For this review, take the finished solid that the model builds, in its own axes (mm). Coordinates: 2 decimals unless noted, no trailing zeros. Order: outer loops, then holes, each group sorted by start corner. A loop starts at its lowest first (then second) coordinate and runs counter-clockwise, first axis right, second up. Notation, with made-up numbers: (13, -36) -> (60, -36) arc R8 cw to (60, -28) -> close; hole circle Ø5 at (73, -24). An arc over 180 degrees is marked (long way). Answer as a JSON object with one key per item and string values. Group by question number.
1) Wall thickness on L1, parallel to Z at x = 10.05, y = 16; L2, parallel to Y at x = 6.85, z = 109.5; L3, parallel to Y at x = 9.05, z = 112: over which ranges is each line inside the solid? List them lowest first.
2) Add section A-A, the plane y = 57.15. Write out the cut boundary in (x, z).
3) Add section B-B, the plane z = 0. Write out the cut boundary in (x, y).
4) Add section C-C, the plane x = 11.3. Count the separate pieces of the cut face and the enclosed holes in it, then the cut area to 3 significant figures.
5) Add section D-D, the plane y = 160. Write out the cut boundary in (x, z).
6) For pin 1 (2 mm diameter, centred on x = 10, y = 144, fed in from -Z); pin 2 (3 mm diameter, centred on x = 10.5, z = 36.5, fed in from -Y); pin 3 (3 mm diameter, centred on x = 9.5, y = 136.5, fed in from -Z), all flat-tipped, find the tip position at first contact; note any pin that passes through.
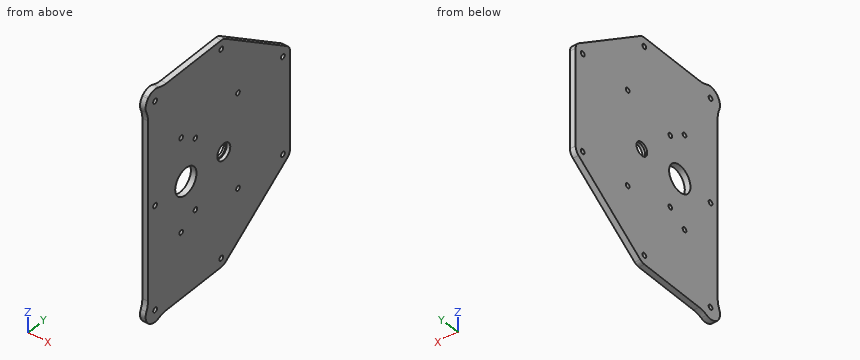
from build123d import *
from build123d.topology import SkipClean

# Parameters (mm, degrees)
ANGLEDBALLAST_DECKFRONT_OUTLINE_R = 2.5527
ANGLEDBALLAST_DECKFRONT_DEPTH     = 6.35
SKETCH1_R                         = 2.5527
BOSS_EXTRUDE1_DEPTH               = 5.9944
SKETCH2_R                         = 7.14375
SKETCH2_R_2                       = 14.2875
CUT_EXTRUDE1_DEPTH                = 344.885135927
F_10_CLEARANCE_HOLE1_AT_2_COUNT   = 2
F_10_CLEARANCE_HOLE1_AT_2_PITCH   = 58.544107304
F_10_CLEARANCE_HOLE1_AT_3_COUNT   = 2
F_10_CLEARANCE_HOLE1_AT_3_PITCH   = 105.685062805
F_10_CLEARANCE_HOLE1_AT_4_COUNT   = 2
F_10_CLEARANCE_HOLE1_AT_4_PITCH   = 76.2
F_10_CLEARANCE_HOLE1_AT_5_COUNT   = 2
F_10_CLEARANCE_HOLE1_AT_5_PITCH   = 90.539312574
F_10_CLEARANCE_HOLE1_AT_6_COUNT   = 2
F_10_CLEARANCE_HOLE1_AT_6_PITCH   = 22.719352983
SKETCH6_R                         = 12.7
SKETCH6_R_2                       = 2.5527
BOSS_EXTRUDE2_DEPTH               = 5.9944
FILLET1_R                         = 25.4
CUT_EXTRUDE2_DEPTH                = 233.633802265
FILLET2_R                         = 9.525
SKETCH8_R                         = 8.73125
CUT_EXTRUDE3_DEPTH                = 3.7846


# Read off the part's stored shape, not the designer's step: Surface Bodies1
with BuildPart() as part:
    # AngledBallast_DeckFront outline → AngledBallast_DeckFront (new body)
    with BuildSketch(Plane.YZ):
        Polygon((227.241295543, 95.25), (0, 257.81), (0, -257.81), (227.241295543, -95.25), align=None)
        with Locations((15.875, -111.125)):
            Circle(ANGLEDBALLAST_DECKFRONT_OUTLINE_R, mode=Mode.SUBTRACT)
        with Locations((104.656174089, -111.125)):
            Circle(ANGLEDBALLAST_DECKFRONT_OUTLINE_R, mode=Mode.SUBTRACT)
        with Locations((187.325, -51.986786112)):
            Circle(ANGLEDBALLAST_DECKFRONT_OUTLINE_R, mode=Mode.SUBTRACT)
        with Locations((15.875, 0)):
            Circle(ANGLEDBALLAST_DECKFRONT_OUTLINE_R, mode=Mode.SUBTRACT)
        with Locations((15.875, 111.125)):
            Circle(ANGLEDBALLAST_DECKFRONT_OUTLINE_R, mode=Mode.SUBTRACT)
        Polygon((101.6, -101.6), (25.4, -101.6), (25.4, 101.6), (101.6, 101.6), (177.8, 47.089344398), (177.8, -47.089344398), align=None, mode=Mode.SUBTRACT)
        with Locations((104.656174089, 111.125)):
            Circle(ANGLEDBALLAST_DECKFRONT_OUTLINE_R, mode=Mode.SUBTRACT)
        with Locations((187.325, 51.986786112)):
            Circle(ANGLEDBALLAST_DECKFRONT_OUTLINE_R, mode=Mode.SUBTRACT)
    extrude(amount=ANGLEDBALLAST_DECKFRONT_DEPTH)


with BuildPart() as body_2:
    # Sketch1 → Boss-Extrude1 (new body)
    with BuildSketch(Plane(origin=(6.35, 0, 0), x_dir=(0, 0, -1), z_dir=(1, 0, 0))):
        Polygon((120.65, 107.712348179), (56.884227826, 196.85), (-56.884227826, 196.85), (-120.65, 107.712348179), (-120.65, 6.35), (120.65, 6.35), align=None)
        with Locations(Location((51.986786112, 187.325, 0), (0, 0, 180))):
            Circle(SKETCH1_R, mode=Mode.SUBTRACT)
        with Locations(Location((111.125, 104.656174089, 0), (0, 0, 180))):
            Circle(SKETCH1_R, mode=Mode.SUBTRACT)
        with Locations(Location((0, 15.875, 0), (0, 0, 180))):
            Circle(SKETCH1_R, mode=Mode.SUBTRACT)
        with Locations(Location((111.125, 15.875, 0), (0, 0, 180))):
            Circle(SKETCH1_R, mode=Mode.SUBTRACT)
        with Locations(Location((-111.125, 15.875, 0), (0, 0, 180))):
            Circle(SKETCH1_R, mode=Mode.SUBTRACT)
        with Locations(Location((-111.125, 104.656174089, 0), (0, 0, 180))):
            Circle(SKETCH1_R, mode=Mode.SUBTRACT)
        with Locations(Location((-51.986786112, 187.325, 0), (0, 0, 180))):
            Circle(SKETCH1_R, mode=Mode.SUBTRACT)
    extrude(amount=BOSS_EXTRUDE1_DEPTH)

    # Sketch2 → Cut-Extrude1 (cut, through all)
    with BuildSketch(Plane(origin=(12.3444, 0, 0), x_dir=(0, 0, -1), z_dir=(1, 0, 0))):
        with Locations((0, 108.0008)):
            Circle(SKETCH2_R)
        with Locations((0, 57.15)):
            Circle(SKETCH2_R_2)
    extrude(amount=-CUT_EXTRUDE1_DEPTH, mode=Mode.SUBTRACT)

    # Sketch5 → #10 Clearance Hole1 (revolve, cut)
    with BuildSketch(Plane(origin=(12.3444, 69.9008, -38.1), x_dir=(0, 0, -1), z_dir=(0, 1, 0))):
        Polygon((0, 0), (0, 13.433662253), (2.4892, 11.938), (2.4892, 0), align=None)
    f_10_clearance_hole1 = revolve(axis=Axis((18.6944, 69.9008, -38.1), (-1, 0, 0)), mode=Mode.SUBTRACT)

    # #10 Clearance Hole1 at 2: #10 Clearance Hole1 ×2
    with Locations(*[Vector(0, 0.9761870601839528, -0.2169304578186562) * (i * F_10_CLEARANCE_HOLE1_AT_2_PITCH) for i in range(1, F_10_CLEARANCE_HOLE1_AT_2_COUNT)]):
        add(f_10_clearance_hole1, mode=Mode.SUBTRACT)

    # #10 Clearance Hole1 at 3: #10 Clearance Hole1 ×2
    with Locations(*[Vector(0, 0.5407575913134985, 0.8411784753765537) * (i * F_10_CLEARANCE_HOLE1_AT_3_PITCH) for i in range(1, F_10_CLEARANCE_HOLE1_AT_3_COUNT)]):
        add(f_10_clearance_hole1, mode=Mode.SUBTRACT)

    # #10 Clearance Hole1 at 4: #10 Clearance Hole1 ×2
    with Locations(*[(0, 0, i * F_10_CLEARANCE_HOLE1_AT_4_PITCH) for i in range(1, F_10_CLEARANCE_HOLE1_AT_4_COUNT)]):
        add(f_10_clearance_hole1, mode=Mode.SUBTRACT)

    # #10 Clearance Hole1 at 5: #10 Clearance Hole1 ×2
    with Locations(*[Vector(0, -0.2109669209657333, 0.9774932011314648) * (i * F_10_CLEARANCE_HOLE1_AT_5_PITCH) for i in range(1, F_10_CLEARANCE_HOLE1_AT_5_COUNT)]):
        add(f_10_clearance_hole1, mode=Mode.SUBTRACT)

    # #10 Clearance Hole1 at 6: #10 Clearance Hole1 ×2
    with Locations(*[Vector(0, -0.8407281674761526, -0.5414574299168776) * (i * F_10_CLEARANCE_HOLE1_AT_6_PITCH) for i in range(1, F_10_CLEARANCE_HOLE1_AT_6_COUNT)]):
        add(f_10_clearance_hole1, mode=Mode.SUBTRACT)

    # Sketch6 → Boss-Extrude2 (add)
    # profile 1 of 2: a face of its own
    with BuildSketch(Plane(origin=(12.3444, 0, 0), x_dir=(0, 0, -1), z_dir=(1, 0, 0))):
        with Locations((-111.125, 15.875)):
            Circle(SKETCH6_R)
        with Locations(Location((-111.125, 15.875, 0), (0, 0, 180))):
            Circle(SKETCH6_R_2, mode=Mode.SUBTRACT)
    # profile 2 of 2: a face of its own
    with BuildSketch(Plane(origin=(12.3444, 0, 0), x_dir=(0, 0, -1), z_dir=(1, 0, 0))):
        with Locations((111.125, 15.875)):
            Circle(SKETCH6_R)
        with Locations(Location((111.125, 15.875, 0), (0, 0, 180))):
            Circle(SKETCH6_R_2, mode=Mode.SUBTRACT)
    extrude(amount=-BOSS_EXTRUDE2_DEPTH)

    # Fillet1
    fillet1_edges = [body_2.edges().sort_by_distance(p)[0] for p in [
        (9.3472, 6.35, 102.724739587),
        (9.3472, 24.275260413, 120.65),
        (9.3472, 6.35, -102.724739587),
        (9.3472, 24.275260413, -120.65),
    ]]
    fillet(fillet1_edges, radius=FILLET1_R)

    # Sketch7 → Cut-Extrude2 (cut, through all)
    with BuildSketch(Plane(origin=(12.3444, 0, 0), x_dir=(0, 0, -1), z_dir=(1, 0, 0))):
        with BuildLine():
            Line((119.525260413, 6.35), (120.65, 6.35))
            Line((120.65, 6.35), (120.65, 7.474739587))
            ThreePointArc((120.65, 7.474739587), (120.105256121, 6.894743879), (119.525260413, 6.35))
        make_face()
        with BuildLine():
            Line((-120.65, 6.35), (-119.525260413, 6.35))
            ThreePointArc((-119.525260413, 6.35), (-120.105256121, 6.894743879), (-120.65, 7.474739587))
            Line((-120.65, 7.474739587), (-120.65, 6.35))
        make_face()
    extrude(amount=-CUT_EXTRUDE2_DEPTH, mode=Mode.SUBTRACT)

    # Fillet2
    fillet2_edges = [body_2.edges().sort_by_distance(p)[0] for p in [
        (9.3472, 107.712348179, 120.65),
        (9.3472, 196.85, 56.884227826),
        (9.3472, 196.85, -56.884227826),
        (9.3472, 107.712348179, -120.65),
    ]]
    fillet(fillet2_edges, radius=FILLET2_R)

    # Sketch8 → Cut-Extrude3 (cut)
    with SkipClean():  # the faces are left unmerged after this step: merging them gives an invalid solid
        with BuildSketch(Plane(origin=(12.3444, 0, 0), x_dir=(0, 0, -1), z_dir=(1, 0, 0))):
            with Locations((0, 108.0008)):
                Circle(SKETCH8_R)
        extrude(amount=-CUT_EXTRUDE3_DEPTH, mode=Mode.SUBTRACT)


solid = body_2.part
Output values:
{
 "1": {"L1": "z = -123.82 to -113.67, -108.58 to -2.55, 2.55 to 108.58, 113.67 to 123.82", "L2": "y = 3.28 to 13.91, 17.84 to 102.69, 106.62 to 123.3", "L3": "y = 3.21 to 13.48, 18.27 to 102.26, 107.05 to 119.8"},
 "2": {"outline": "(6.35, -120.65) -> (12.34, -120.65) -> (12.34, -14.29) -> (6.35, -14.29) -> close; (6.35, 14.29) -> (12.34, 14.29) -> (12.34, 120.65) -> (6.35, 120.65) -> close"},
 "3": {"outline": "(6.35, 6.35) -> (12.34, 6.35) -> (12.34, 13.32) -> (6.35, 13.32) -> close; (6.35, 18.43) -> (12.34, 18.43) -> (12.34, 42.86) -> (6.35, 42.86) -> close; (6.35, 71.44) -> (12.34, 71.44) -> (12.34, 99.27) -> (8.56, 99.27) -> (8.56, 100.86) -> (6.35, 100.86) -> close; (6.35, 115.14) -> (8.56, 115.14) -> (8.56, 116.73) -> (12.34, 116.73) -> (12.34, 196.85) -> (6.35, 196.85) -> close"},
 "4": {"separate pieces": "1", "enclosed holes": "15", "area": "39,300 mm²"},
 "5": {"outline": "(6.35, -83.25) -> (12.34, -83.25) -> (12.34, 83.25) -> (6.35, 83.25) -> close"},
 "6": {"pin 1": "stops at z = -95.41", "pin 2": "stops at y = 6.35", "pin 3": "stops at z = -101.13"}
}
